Here's how the part is built. I have some questions about the finished solid (model axes, mm). A direction names the side the tool comes from. Coordinates: 2 decimals unless noted, no trailing zeros. Order: outer loops, then holes, each group sorted by start corner. A loop starts at its lowest first (then second) coordinate and runs counter-clockwise, first axis right, second up. Notation, with made-up numbers: M 45,49.5 L 75,49.5 A18 ccw 75,55.5 Z; hole C 13.5,68.5 d3. An arc over 180 degrees is marked long. Answer as CSV lines item,"result". Start each with the question number.
```python
from build123d import *

# Parameters (mm, degrees)
SKETCH1_W           = 4.3
SKETCH1_H           = 15.2
BOSS_EXTRUDE1_DEPTH = 5
SKETCH2_W           = 2
SKETCH2_H           = 10.7
CUT_EXTRUDE1_DEPTH  = 2
SKETCH3_R           = 0.225
BOSS_EXTRUDE2_DEPTH = 4


with BuildPart() as part:
    # Sketch1 → Boss-Extrude1 (new body)
    with BuildSketch(Plane.XY):
        with Locations((2.15, 7.6)):
            Rectangle(SKETCH1_W, SKETCH1_H)
    extrude(amount=BOSS_EXTRUDE1_DEPTH)

    # Sketch2 → Cut-Extrude1 (cut)
    with BuildSketch(Plane(origin=(4.3, 0, 0), x_dir=(0, 0, -1), z_dir=(1, 0, 0))):
        with Locations((-2.5, 8.35)):
            Rectangle(SKETCH2_W, SKETCH2_H)
    extrude(amount=-CUT_EXTRUDE1_DEPTH, mode=Mode.SUBTRACT)

    # Sketch3 → Boss-Extrude2 (add)
    with BuildSketch(Plane.XZ):
        with Locations((1.7, 1.23)):
            Circle(SKETCH3_R)
        with Locations((1.7, 3.77)):
            Circle(SKETCH3_R)
    extrude(amount=BOSS_EXTRUDE2_DEPTH)


solid = part.part
```
1) Suppose I cut it at A-A on x = 4. Please give me the cut outline in (y, z), plus the area to 3 significant figures.
2) Suppose I cut it at C-C on x = 1.7. Please give me the cut outline in (y, z) (3 decimals), plus the area to 3 significant figures.
3) I need wall thicknesses on line 1 (Y direction, x = 3.6, z = 3.05); line 2 (Z direction, x = 3.85, y = 13); line 3 (Y direction, x = 4.05, z = 4.6). Which ranges of each line are inside material? Lowest first, please. Write a range as [from, to].
4) Will these pins go through, and if not, where does the flat tip stop? pin 1 Ø1.5 at (x, z) = (2.5, 2) entering from -Y; pin 2 Ø1 at (y, z) = (6.5, 2.5) entering from +X; pin 3 Ø1.5 at (x, y) = (2, -1.5) entering from +Z (3 decimals).
5) Suppose I cut it at B-B on y = -0.5. Please give me the cut outline in (x, z) (3 decimals), plus the area to 3 significant figures.
6) Which directions (+Z, -Z, +X, -X, +Y, -Y) give clear straight access to the entire face, cutting with the end or side of a thin tool? Please do faces 1 (the face through (3, 8, 1.5)), 2 (the face through (0, 7, 2)).
7) Suppose I cut it at D-D on z = 1.23. Please give me the cut outline in (x, y) (3 decimals).
8) If we mould it in two halves opening along Y, with no side actions, what happens to faces 3 (the face through (2, 15.2, 2)), 4 (the face through (2, 8, 5)), 5 (the face through (3, 3, 3))? For each: released by +Y, released by -Y, zero draft, split by the parting line, or undercut.
Output:
1,outline,"M 0,0 L 15.2,0 L 15.2,5 L 0,5 Z; hole M 3,1.5 L 13.7,1.5 L 13.7,3.5 L 3,3.5 Z"
1,area,"54.6 mm²"
2,outline,"M -4,1.005 L 0,1.005 L 0,0 L 15.2,0 L 15.2,5 L 0,5 L 0,3.995 L -4,3.995 L -4,3.545 L 0,3.545 L 0,1.455 L -4,1.455 Z"
2,area,"79.6 mm²"
3,line 1,"[0, 3], [13.7, 15.2]"
3,line 2,"[0, 1.5], [3.5, 5]"
3,line 3,"[0, 15.2]"
4,pin 1,"y = 0"
4,pin 2,"x = 2.3"
4,pin 3,"z = 3.995"
5,outline,"C 1.7,1.23 d0.45; C 1.7,3.77 d0.45"
5,area,"0.318 mm²"
6,face 1,"+X"
6,face 2,"+Z, -Z, -X, +Y, -Y"
7,outline,"M 0,0 L 1.475,0 L 1.475,-4 L 1.925,-4 L 1.925,0 L 4.3,0 L 4.3,15.2 L 0,15.2 Z"
8,face 3,"released by +Y"
8,face 4,"zero draft"
8,face 5,"undercut"
